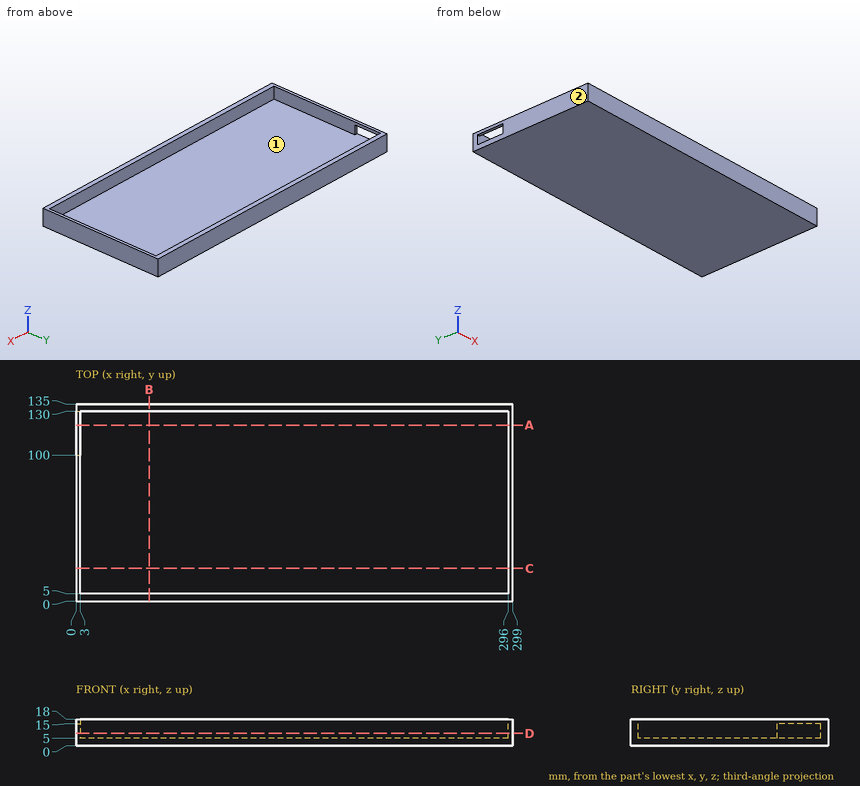
Design review of the part shown in the three views and the two pictorial views. Dimensions are in mm from the part's minimum x, y and z. Give positions to 0.01 mm unless a question says otherwise; leave off trailing zeros. Write each loop counter-clockwise with the first axis right and the second up, starting at its lowest first coordinate (ties: lowest second). Pieces come first, ordered by that corner, then holes. Notation, with made-up numbers: M 46,52.5 L 98,52.5 A29 ccw 98,78.5 Z; hole C -37,49 d10. An arc over 180 degrees is marked long. Return JSON: item names as keys, results as strings. Group by question number.
Item 1: Take a section at A-A (y = 120.5). Give the boundary of the cut face in (x, z).
Item 2: The part is to be moulded in two halves that separate along Y. For the marked faces 1 and 2, say which applies: pulls with the +Y half, pulls with the -Y half, needs draft (parallel to the pull), parting line crosses it, or undercut.
Item 3: Take a section at B-B (x = 50). Give the boundary of the cut face in (y, z), plus the area to 3 significant figures.
Item 4: Clearance check with a flat-ended pin moving along its axis: pin 1 Ø2 at (x, y) = (138.5, 112) entering from +Z. State where the tip first meets the part, or that it passes through.
Item 5: Take a section at C-C (y = 22.5). Give the boundary of the cut face in (x, z), plus the area to 3 significant figures.
Item 6: Wall thickness on line 1 along Y through (x, z) = (231, 13.5); line 2 along X through (y, z) = (113.5, 17); line 3 along Z through (x, y) = (128.5, 70): over which ranges is each line inside the solid? List them lowest first.
Item 7: Take a section at D-D (z = 8.25). Give the boundary of the cut face in (x, y).
Return value:
{
 "1": {"outline": "M 0,0 L 299,0 L 299,18 L 296,18 L 296,5 L 0,5 Z; M 0,15 L 3,15 L 3,18 L 0,18 Z"},
 "2": {"face 1": "undercut", "face 2": "needs draft"},
 "3": {"outline": "M 0,0 L 135,0 L 135,18 L 130,18 L 130,5 L 5,5 L 5,18 L 0,18 Z", "area": "805 mm2"},
 "4": {"pin 1": "stops at z = 5"},
 "5": {"outline": "M 0,0 L 299,0 L 299,18 L 296,18 L 296,5 L 3,5 L 3,18 L 0,18 Z", "area": "1,570 mm2"},
 "6": {"line 1": "y = 0 to 5, 130 to 135", "line 2": "x = 0 to 3, 296 to 299", "line 3": "z = 0 to 5"},
 "7": {"outline": "M 0,0 L 299,0 L 299,135 L 0,135 L 0,130 L 296,130 L 296,5 L 3,5 L 3,100 L 0,100 Z"}
}
